Here's how the part is built. I have some questions about the finished solid (model axes, mm). Face numbers are marked on the shaded views. A direction names the side the tool comes from. Give positions to 0.01 mm unless a question says otherwise; leave off trailing zeros. Loops run counter-clockwise (first coordinate to the right, second up) from the corner with the lowest first, then second, coordinate; pieces in that order, holes last. Notation, with made-up numbers: (-9.75, 67) - (4.25, 67) arc R27 ccw to (4.25, 90) - close; hole circle Ø8 at (-17, 40.25). An arc over 180 degrees is marked (long way). Return JSON: item names as keys, results as strings. Group by question number.
(1) If we section it at D-D (y = -3.25): Please give me the cut outline in (x, z).
(2) If we section it at C-C (z = 7): Please give me the cut outline in (x, y).
(3) If we section it at B-B (y = 0): Please give me the cut outline in (x, z), then the cut area to 3 significant figures.
(4) If we mould it in two halves opening along Y, with no side actions, what happens to the marked faces 1 and 2? For each: released by +Y, released by -Y, zero draft, split by the parting line, or undercut.
(5) I need wall thicknesses on probe 1 along Z at (x, y) = (0.75, 5.5); probe 2 along Z at (x, y) = (0.75, 0.25); probe 3 along Y at (x, z) = (0.5, 3.5). Which ranges of each line are inside material? Lowest first, please. Write a range as [from, to].
(6) On a 3-axis mill with a long thin cutter (end or side, diameter ignored), from which of +Z, -Z, +X, -X, +Y, -Y can I reach the whole of each face in a straight line? I mean the marked faces 3 and 4. Say none if no direction works.
(7) If we section it at A-A (x = 0): Please give me the cut outline in (y, z).
(8) For P1, Ø5, axis at y = -0.5, z = 12, coming from the +X side; P2, Ø2, axis at y = 4.5, z = 12, coming from the +X side; P3, Ø6, axis at x = 4, z = 14, coming from the -Y side, each with a flat end and sliding along its axis, tell me the tip position at first contact or that it passes through.
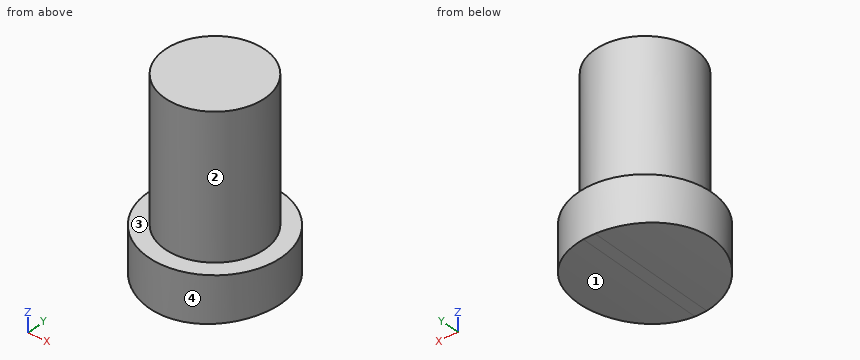
```python
from build123d import *

# Parameters (mm, degrees)
SKETCH1_R           = 4.5
BOSS_EXTRUDE1_DEPTH = 17
SKETCH1_4_R         = 6
SKETCH1_4_R_2       = 4.5
BOSS_EXTRUDE2_DEPTH = 4.25
CUT_EXTRUDE1_DEPTH  = 6


with BuildPart() as part:
    # Sketch1 → Boss-Extrude1 (new body)
    with BuildSketch(Plane.XY):
        Circle(SKETCH1_R)
    extrude(amount=BOSS_EXTRUDE1_DEPTH)

    # Sketch1<4> → Boss-Extrude2 (add)
    with BuildSketch(Plane.XY):
        Circle(SKETCH1_4_R)
        Circle(SKETCH1_4_R_2, mode=Mode.SUBTRACT)
    extrude(amount=BOSS_EXTRUDE2_DEPTH)

    # Sketch2 → Cut-Extrude1 (cut, symmetric)
    with BuildSketch(Plane(origin=(0, 0, 0), x_dir=(1, 0, 0), z_dir=(0, 1, 0))):
        with BuildLine():
            Line((-6, 0), (-6, -0.37451045))
            ThreePointArc((-6, -0.37451045), (-3.27018436, -0.108880819), (-0.529637427, 0))
            Line((-0.529637427, 0), (-6, 0))
        make_face()
        with BuildLine():
            Line((6, 0), (0.529637427, 0))
            ThreePointArc((0.529637427, 0), (3.27018436, -0.108880819), (6, -0.37451045))
            Line((6, -0.37451045), (6, 0))
        make_face()
    extrude(amount=CUT_EXTRUDE1_DEPTH, both=True, mode=Mode.SUBTRACT)


solid = part.part
```
Values:
{
 "1": {"outline": "(-5.04, 0.26) arc R47.88 ccw to (-0.53, 0) - (0.53, 0) arc R47.88 ccw to (5.04, 0.26) - (5.04, 4.25) - (3.11, 4.25) - (3.11, 17) - (-3.11, 17) - (-3.11, 4.25) - (-5.04, 4.25) - close"},
 "2": {"outline": "circle Ø9 at (0, 0)"},
 "3": {"outline": "(-6, 0.37) arc R47.88 ccw to (-0.53, 0) - (0.53, 0) arc R47.88 ccw to (6, 0.37) - (6, 4.25) - (4.5, 4.25) - (4.5, 17) - (-4.5, 17) - (-4.5, 4.25) - (-6, 4.25) - close", "area": "164 mm2"},
 "4": {"face 1": "zero draft", "face 2": "split by the parting line"},
 "5": {"probe 1": "[0, 4.25]", "probe 2": "[0, 17]", "probe 3": "[-5.98, 5.98]"},
 "6": {"face 3": "+Z", "face 4": "+Z, -Z"},
 "7": {"outline": "(-6, 0) - (6, 0) - (6, 4.25) - (4.5, 4.25) - (4.5, 17) - (-4.5, 17) - (-4.5, 4.25) - (-6, 4.25) - close"},
 "8": {"P1": "x = 4.5", "P2": "x = 2.83", "P3": "y = -4.39"}
}
